The model under review builds one solid part; all positions refer to its coordinate system, in mm. Face numbers are marked on the shaded views. Give positions to 0.01 mm unless a question says otherwise; leave off trailing zeros. Loops run counter-clockwise (first coordinate to the right, second up) from the corner with the lowest first, then second, coordinate; pieces in that order, holes last. Notation, with made-up numbers: (-27, 15) - (4, 15) arc R35 cw to (4, 53) - close; hole circle Ø9 at (-11.75, -31). An arc over 180 degrees is marked (long way). Answer as a JSON object with one key per item and string values.
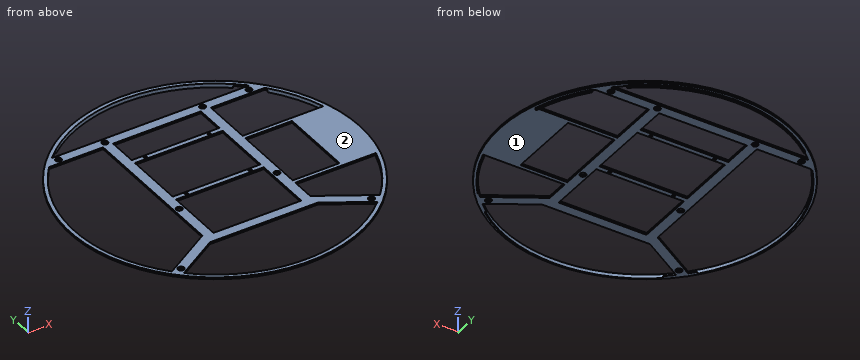
from build123d import *

# Parameters (mm, degrees)
SKIZZE1_R                = 72.5
SKIZZE1_R_2              = 70.5
BASE_RING_DEPTH          = 1
SKIZZE2_W                = 22
SKIZZE2_H                = 2.5
RASPBERRY_FRAME_DEPTH    = 1
SCREWS_I_D               = 3
FAN_SCREWS_D             = 1.5
TOP_START                = -1
SKIZZE7_W                = 23.5
SKIZZE7_H                = 2
TOP_COVER_DEPTH          = 1
INNER_START              = 1
INNER_RING_DEPTH         = 1
LOWER_COVER_CUT_DEPTH    = 103.535359755
COVER_CUT_ROTATION_COUNT = 4


with BuildPart() as part:
    # Skizze1 → Base Ring (new body)
    with BuildSketch(Plane.XY):
        Circle(SKIZZE1_R)
        Circle(SKIZZE1_R_2, mode=Mode.SUBTRACT)
    extrude(amount=BASE_RING_DEPTH)

    # Skizze2 → Raspberry Frame (add)
    with BuildSketch(Plane.XY):
        with BuildLine():
            Line((0, 50.22970773), (-49.469449778, 50.22970773))
            ThreePointArc((-49.469449778, 50.22970773), (-51.834480078, 47.785318614), (-54.078864066, 45.22970773))
            Line((-54.078864066, 45.22970773), (-27, 45.22970773))
            Line((-27, 45.22970773), (-22, 45.22970773))
            Line((-22, 45.22970773), (0, 45.22970773))
            Line((0, 45.22970773), (0, 50.22970773))
        make_face()
        Polygon((-22, 45.22970773), (-27, 45.22970773), (-27, -32.164435383), (-27, -33.02029227), (-22, -33.02029227), (-22, -3.77029227), (-22, -1.27029227), (-22, 28.22970773), (-22, 30.72970773), align=None)
        with BuildLine():
            Line((-27, -32.164435383), (-52.117379441, -47.476612771))
            ThreePointArc((-52.117379441, -47.476612771), (-50.354632641, -49.34228381), (-48.5251414, -51.142552264))
            Line((-48.5251414, -51.142552264), (-27, -38.02029227))
            Line((-27, -38.02029227), (-27, -33.02029227))
            Line((-27, -33.02029227), (-27, -32.164435383))
        make_face()
        Polygon((-27, -33.02029227), (-27, -38.02029227), (0, -38.02029227), (0, -33.02029227), (-22, -33.02029227), align=None)
        with Locations((-11, 29.47970773)):
            Rectangle(SKIZZE2_W, SKIZZE2_H)
        with Locations((-11, -2.52029227)):
            Rectangle(SKIZZE2_W, SKIZZE2_H)
    raspberry_frame = extrude(amount=RASPBERRY_FRAME_DEPTH)

    # Screws I (through all)
    with Locations(Plane.XY.offset(1)):
        with Locations((-47.72970773, -47.72970773), (-24.5, -10.27029227), (-47.72970773, 47.72970773), (-24.5, 47.72970773)):
            screws_i = Hole(SCREWS_I_D / 2)

    # Fan Screws (through all)
    with Locations(Plane.XY.offset(1)):
        with Locations((-16, 29.47970773), (-16, -2.52029227)):
            fan_screws = Hole(FAN_SCREWS_D / 2)

    # Mirror I: Raspberry Frame, Screws I, Fan Screws across plane
    add(raspberry_frame.mirror(Plane(origin=(0, 0, 0), x_dir=(0, 0, 1), z_dir=(1, 0, 0))))
    add(screws_i.mirror(Plane(origin=(0, 0, 0), x_dir=(0, 0, 1), z_dir=(1, 0, 0))), mode=Mode.SUBTRACT)
    add(fan_screws.mirror(Plane(origin=(0, 0, 0), x_dir=(0, 0, 1), z_dir=(1, 0, 0))), mode=Mode.SUBTRACT)

    # Skizze7 → Top Cover (add)
    with BuildSketch(Plane.XY.offset(1).offset(TOP_START)):
        with BuildLine():
            Line((50.5, -18.5), (50.5, -20.5))
            Line((50.5, -20.5), (67.453687816, -20.5))
            ThreePointArc((67.453687816, -20.5), (69.734263426, -10.36255299), (70.5, 0))
            ThreePointArc((70.5, 0), (69.734263426, 10.36255299), (67.453687816, 20.5))
            Line((67.453687816, 20.5), (50.5, 20.5))
            Line((50.5, 20.5), (50.5, 18.5))
            Line((50.5, 18.5), (50.5, -18.5))
        make_face()
        with Locations((38.75, 19.5)):
            Rectangle(SKIZZE7_W, SKIZZE7_H)
        with Locations((38.75, -19.5)):
            Rectangle(SKIZZE7_W, SKIZZE7_H)
    extrude(amount=TOP_COVER_DEPTH)

    # Skizze8 → Inner Ring (add)
    with BuildSketch(Plane(origin=(0, 0, 0), x_dir=(-1, 0, 0), z_dir=(0, 0, -1)).offset(INNER_START)):
        with BuildLine():
            Line((-67.976098741, 20.5), (-67.453687816, 20.5))
            ThreePointArc((-67.453687816, 20.5), (70.5, 0), (-67.453687816, -20.5))
            Line((-67.453687816, -20.5), (-67.976098741, -20.5))
            ThreePointArc((-67.976098741, -20.5), (71, 0), (-67.976098741, 20.5))
        make_face()
    extrude(amount=-INNER_RING_DEPTH)

    # Skizze9 → Lower Cover Cut (cut, through all)
    with BuildSketch(Plane(origin=(0, 0, 0), x_dir=(-1, 0, 0), z_dir=(0, 0, -1))):
        Polygon((-45.961940777, -56.568542495), (-38.890872965, -49.497474683), (-49.497474683, -38.890872965), (-56.568542495, -45.961940777), align=None)
    lower_cover_cut = extrude(amount=LOWER_COVER_CUT_DEPTH, mode=Mode.SUBTRACT)

    # Cover Cut Rotation: Lower Cover Cut ×4 about axis
    cover_cut_rotation_axis = Axis((0, 0, 0), (0, 0, 1))
    for i in range(1, COVER_CUT_ROTATION_COUNT):
        add(lower_cover_cut.rotate(cover_cut_rotation_axis, i * 360 / COVER_CUT_ROTATION_COUNT), mode=Mode.SUBTRACT)


solid = part.part
Q1. To check wall thickness, follow probe 1 along X at (y, z) = (-29.5, 0.8); probe 2 along Y at (x, z) = (-5.5, 0.8); probe 3 along X at (y, z) = (-9, 0.75). State the ranges of each line that lie inside material, in increasing order. Write a range as [from, to].
Results:
{"probe 1": "x = [-66.23, -64.03], [-27, -22], [22, 27], [64.03, 66.23]", "probe 2": "y = [-72.29, -70.29], [-38.02, -33.02], [-3.77, -1.27], [28.23, 30.73], [45.23, 50.23], [70.29, 72.29]", "probe 3": "x = [-71.94, -69.92], [-27, -25.3], [-23.7, -22], [22, 23.7], [25.3, 27], [50.5, 71.94]"}
Q2. Consider section A-A, the plane x = 0. State the section outline as (y, z) points, plus the area to 3 significant figures.
Results:
{"outline": "(-72.5, 0) - (-71, 0) - (-71, -1) - (-70.5, -1) - (-70.5, 1) - (-72.5, 1) - close; (-38.02, 0) - (-33.02, 0) - (-33.02, 1) - (-38.02, 1) - close; (-3.77, 0) - (-1.27, 0) - (-1.27, 1) - (-3.77, 1) - close; (28.23, 0) - (30.73, 0) - (30.73, 1) - (28.23, 1) - close; (45.23, 0) - (50.23, 0) - (50.23, 1) - (45.23, 1) - close; (70.5, -1) - (71, -1) - (71, 0) - (72.5, 0) - (72.5, 1) - (70.5, 1) - close", "area": "20.0 mm^2"}
Q3. The part is to be moulded in two halves that separate along Y. For the marked faces 1 and 2, say which applies: +Y half, -Y half, draft (parallel to the pull), parting line (faces both ways), or undercut.
Results:
{"face 1": "undercut", "face 2": "draft"}
Q4. Clearance check with flat-ended pins moving along their axes: pin 1 Ø0.5 at (x, z) = (-8.5, 0.5) entering from -Y; pin 2 Ø1.1 at (x, z) = (3.5, 0.5) entering from +Y; pin 3 Ø0.5 at (x, z) = (6.5, 0.5) entering from +Y; pin 4 Ø0.9 at (x, y) = (-16, 29.48) entering from -Z. State where each tip first meets the part, or that it passes through.
Results:
{"pin 1": "stops at y = -72.03", "pin 2": "stops at y = 72.44", "pin 3": "stops at y = 72.23", "pin 4": "passes through"}
Q5. Consider section B-B, the plane y = 26. State the section outline as (x, z) points, plus the area to 3 significant figures.
Results:
{"outline": "(-67.68, 0) - (-66.07, 0) - (-66.07, -1) - (-65.53, -1) - (-65.53, 1) - (-67.68, 1) - close; (-27, 0) - (-22, 0) - (-22, 1) - (-27, 1) - close; (22, 0) - (27, 0) - (27, 1) - (22, 1) - close; (65.53, -1) - (66.07, -1) - (66.07, 0) - (67.68, 0) - (67.68, 1) - (65.53, 1) - close", "area": "15.4 mm^2"}
Q6. Consider section D-D, the plane y = -40. State the section outline as (x, z) points, plus the area to 3 significant figures.
Results:
{"outline": "(-60.47, 0) - (-58.66, 0) - (-58.66, -1) - (-58.05, -1) - (-58.05, 1) - (-60.47, 1) - close; (-39.85, 0) - (-30.25, 0) - (-30.25, 1) - (-39.85, 1) - close; (30.25, 0) - (39.85, 0) - (39.85, 1) - (30.25, 1) - close; (58.05, -1) - (58.66, -1) - (58.66, 0) - (60.47, 0) - (60.47, 1) - (58.05, 1) - close", "area": "25.2 mm^2"}
Q7. Consider section C-C, the plane z = 0.45. State how many separate pieces and enclosed holes the cut face has, plus the area to 3 significant figures.
Results:
{"separate pieces": "1", "enclosed holes": "21", "area": "3,770 mm^2"}
